CAD build for the part. Positions are in the model's coordinates, mm. Face numbers are marked on the shaded views. A direction names the side the tool comes from. Round coordinates to 2 decimals unless told otherwise and drop trailing zeros. Loops run counter-clockwise (first coordinate to the right, second up) from the corner with the lowest first, then second, coordinate; pieces in that order, holes last.
from build123d import *

# Parameters (mm, degrees)
SKETCH1_R           = 2
BOSS_EXTRUDE1_DEPTH = 2.5
FILLET1_R           = 0.1
SKETCH2_R           = 4.5
SKETCH2_R_2         = 2
BOSS_EXTRUDE2_DEPTH = 1
FILLET2_R           = 0.1


with BuildPart() as part:
    # Sketch1 → Boss-Extrude1 (new body)
    with BuildSketch(Plane(origin=(0, 0, 0), x_dir=(1, 0, 0), z_dir=(0, 1, 0))):
        Polygon((2.020725942, -3.5), (4.041451884, 0), (2.020725942, 3.5), (-2.020725942, 3.5), (-4.041451884, 0), (-2.020725942, -3.5), align=None)
        with Locations(Location((0, 0, 0), (0, 0, 270))):
            Circle(SKETCH1_R, mode=Mode.SUBTRACT)
    extrude(amount=BOSS_EXTRUDE1_DEPTH)

    # Fillet1
    fillet1_edges = [part.edges().sort_by_distance(p)[0] for p in [
        (3.031088913, 2.5, -1.75),
        (0, 2.5, -3.5),
        (-3.031088913, 2.5, -1.75),
        (0, 0, -2),
        (0, 2.5, -2),
        (-3.031088913, 2.5, 1.75),
        (0, 2.5, 3.5),
        (-3.031088913, 0, 1.75),
        (-3.031088913, 0, -1.75),
        (0, 0, -3.5),
        (3.031088913, 2.5, 1.75),
        (3.031088913, 0, -1.75),
        (3.031088913, 0, 1.75),
        (0, 0, 3.5),
    ]]
    fillet(fillet1_edges, radius=FILLET1_R)

    # Sketch2 → Boss-Extrude2 (add)
    with BuildSketch(Plane(origin=(0, 2.5, 0), x_dir=(1, 0, 0), z_dir=(0, 1, 0))):
        with Locations(Location((0, 0, 0), (0, 0, 270))):
            Circle(SKETCH2_R)
        with Locations(Location((0, 0, 0), (0, 0, 270))):
            Circle(SKETCH2_R_2, mode=Mode.SUBTRACT)
    extrude(amount=BOSS_EXTRUDE2_DEPTH)

    # Fillet2
    fillet2_edges = [part.edges().sort_by_distance(p)[0] for p in [
        (0, 3.5, -4.5),
        (0, 2.5, -4.5),
        (0, 3.5, -2),
    ]]
    fillet(fillet2_edges, radius=FILLET2_R)


solid = part.part
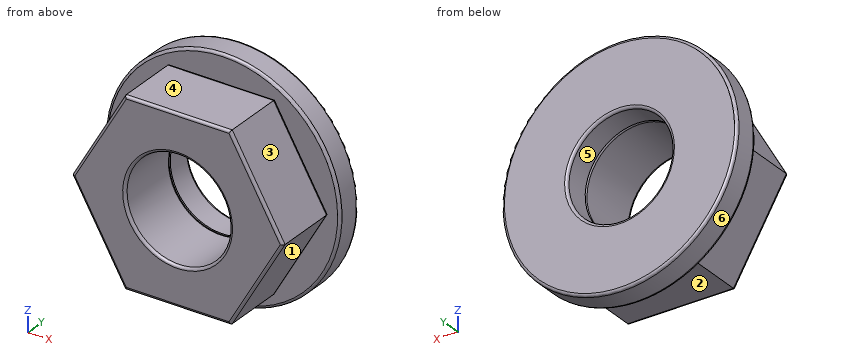
Item 1: Mould opens along Z. For the marked faces 4, 5 and 6 say: released by +Z, released by -Z, zero draft, split by the parting line, or undercut.
Verdict:
face 4: released by +Z
face 5: undercut
face 6: split by the parting line
Item 2: Wall check: L1, parallel to X at y = 2.8, z = 0; L2, parallel to Y at x = -3.5, z = 2; L3, parallel to Z at x = 1, y = 1.65. Give the ranges that are in metal, low to high.
Verdict:
L1: x = -4.5 to -2, 2 to 4.5
L2: y = 2.5 to 3.5
L3: z = -3.5 to -1.73, 1.73 to 3.5
Item 3: 3-axis set-ups, long thin cutter, end or side, ignore diameter. For the marked faces 1, 2 and 3: which of +Z, -Z, +X, -X, +Y, -Y reach the whole face in a straight line?
Verdict:
face 1: -Z, +X, -Y
face 2: -Z, +X, -X, -Y
face 3: +Z, +X, -Y
Item 4: Cut at B-B (y = 0.8). List the corners of the cut face in (x, z).
Verdict:
outline: (-4.04, 0) - (-2.02, -3.5) - (2.02, -3.5) - (4.04, 0) - (2.02, 3.5) - (-2.02, 3.5) - close; hole circle Ø4 at (0, 0)
Item 5: Flat gauge pins, fed straight in: P1, Ø2.5, axis at x = 0, z = 0, coming from the -Y side; P2, Ø1.2, axis at x = -0.5, y = 1.5, coming from the +Z side; P3, Ø0.7, axis at x = 0, y = 1, coming from the -Z side; P4, Ø1, axis at x = -1, y = 2.5, coming from the +Z side. Where does each tip first touch, or does it go through?
Verdict:
P1: passes through
P2: stops at z = 3.5
P3: stops at z = -3.5
P4: stops at z = 4.47
